Design review of the part shown in the three views and the two pictorial views. Dimensions are in mm from the part's minimum x, y and z. A direction names the side the tool comes from. Round coordinates to 2 decimals unless told otherwise and drop trailing zeros. Order: outer loops, then holes, each group sorted by start corner. A loop starts at its lowest first (then second) coordinate and runs counter-clockwise, first axis right, second up. Notation, with made-up numbers: (-7, 83.25) -> (17, 83.25) arc R24 cw to (17, 98.25) -> close; hole circle Ø10 at (85.25, 75.5). An arc over 180 degrees is marked (long way). Put each result on its own line as item: value. Start each with the question number.
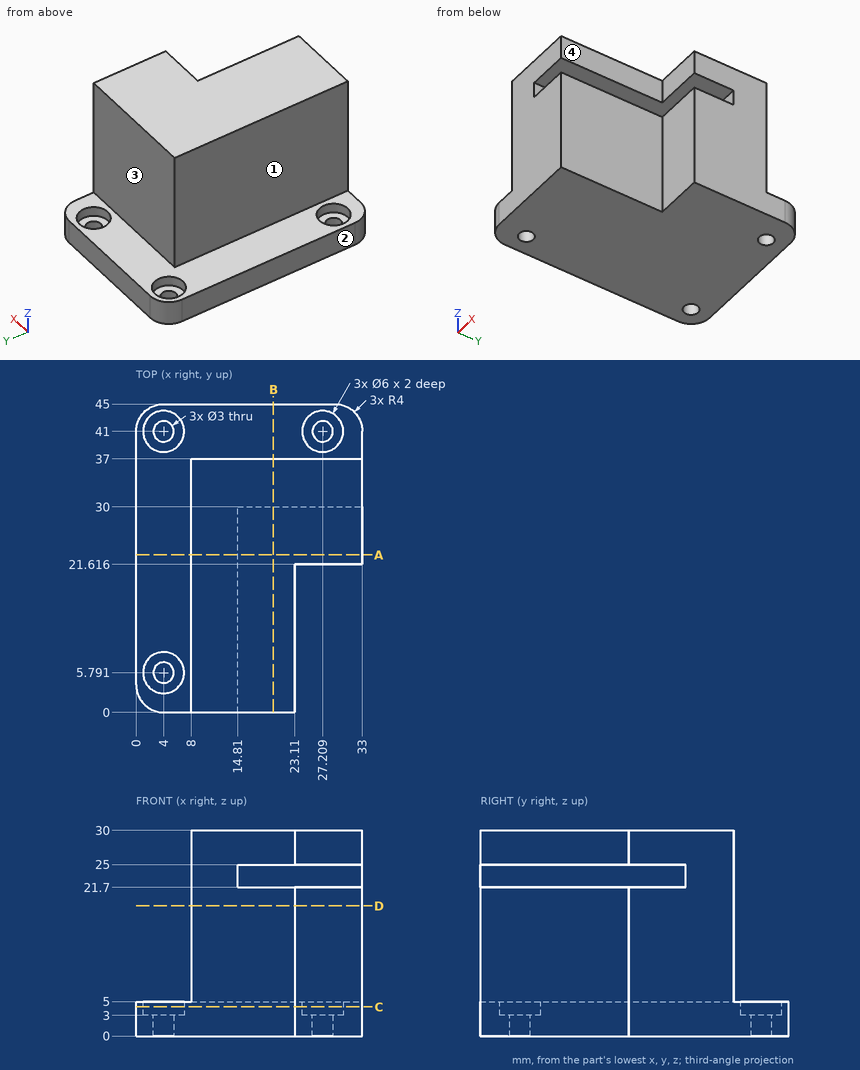
Q1. Take a section at B-B on x = 20. Give the boundary of the cut face in (y, z), and give its area (3 significant figures).
Q2. Wall thickness on probe 1 along Y at (x, z) = (4, 3.6); probe 2 along X at (y, z) = (41, 3.85); probe 3 along Y at (x, z) = (4, 2.25): over which ranges is each line inside the solid? List them lowest first. Write a range as [from, to].
Q3. Take a section at C-C on z = 4.25. Give the boundary of the cut face in (x, y), and give its area (3 significant figures).
Q4. Clearance check with flat-ended pins moving along their axes: pin 1 Ø6.5 at (x, y) = (4, 7) entering from +Z; pin 2 Ø3 at (x, y) = (28, 42) entering from +Z; pin 3 Ø2.5 at (y, z) = (8, 27) entering from +X. State where each tip first meets the part, or that it passes through.
Q5. Take a section at A-A on y = 23. Give the boundary of the cut face in (x, z), and give its area (3 significant figures).
Q6. For the marked faces 1, 2, 3 and 4, list the 3-axis set-ups (+Z, -Z, +X, -X, +Y, -Y) from which the entire face can be reached by the end or side of a thin tool; tool diameter is ignored.
Q7. Take a section at D-D on z = 19. Give the boundary of the cut face in (x, y).
Calculated:
1. outline: (0, 0) -> (45, 0) -> (45, 5) -> (37, 5) -> (37, 30) -> (0, 30) -> (0, 25) -> (30, 25) -> (30, 21.7) -> (0, 21.7) -> close
1. area: 1,050 mm²
2. probe 1: y = [0, 2.79], [8.79, 38], [44, 45]
2. probe 2: x = [0, 1], [7, 24.21], [30.21, 33]
2. probe 3: y = [0, 4.29], [7.29, 39.5], [42.5, 45]
3. outline: (0, 4) arc R4 ccw to (4, 0) -> (23.11, 0) -> (23.11, 21.62) -> (33, 21.62) -> (33, 41) arc R4 ccw to (29, 45) -> (4, 45) arc R4 ccw to (0, 41) -> close; hole circle Ø6 at (4, 5.79); hole circle Ø6 at (4, 41); hole circle Ø6 at (27.21, 41)
3. area: 1,180 mm²
4. pin 1: stops at z = 5
4. pin 2: stops at z = 3
4. pin 3: stops at x = 23.11
5. outline: (0, 0) -> (33, 0) -> (33, 21.7) -> (14.81, 21.7) -> (14.81, 25) -> (33, 25) -> (33, 30) -> (8, 30) -> (8, 5) -> (0, 5) -> close
5. area: 730 mm²
6. face 1: +Z, -X, +Y, -Y
6. face 2: +Z, -Z, -X, +Y, -Y
6. face 3: +Z, +X, -X, +Y
6. face 4: +Z, -Z, +X, -Y
7. outline: (8, 0) -> (23.11, 0) -> (23.11, 21.62) -> (33, 21.62) -> (33, 37) -> (8, 37) -> close
